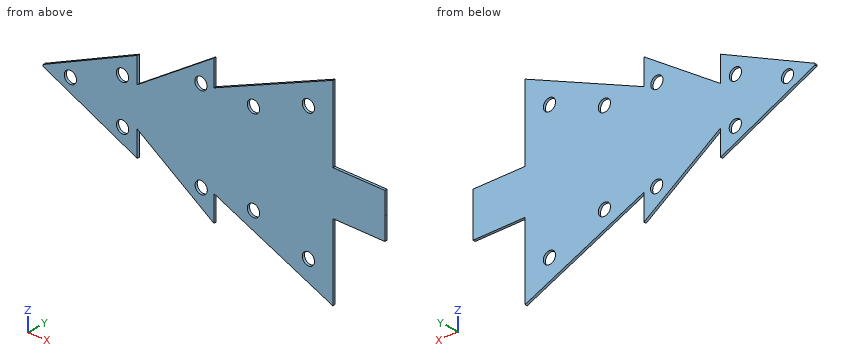
Autodesk Inventor part; units mm, degrees
ref_plane "YZ Plane" through (0, 0, 0) normal (1, 0, 0) x (0, 1, 0)
ref_plane "XZ Plane" through (0, 0, 0) normal (0, 1, 0) x (-1, 0, 0)
ref_plane "XY Plane" through (0, 0, 0) normal (0, 0, 1) x (1, 0, 0)
sketch "Sketch1" plane through (0, 0, 0) normal (0, 1, 0) x (-1, 0, 0)
  line L0 (-128.7932, -21.9318) -> (-128.8163, -31.0141)
  line L1 (11.205, -31.37) -> (11.2067, -30.7124)
  line L2 (11.2067, -30.7124) -> (-27.3951, -12.7346)
  line L3 (-27.3951, -12.7346) -> (-27.3951, -23.154)
  line L4 (-27.3951, -23.154) -> (-58.7933, -1.6646)
  line L5 (-58.7933, -1.6646) -> (-58.7933, -12.2738)
  line L6 (-58.7933, -12.2738) -> (-107.4995, 9.0183)
  line L7 (-107.4995, 9.0183) -> (-107.4995, -21.9859)
  line L8 (-107.4995, -21.9859) -> (-128.7932, -21.9318)
  line L9 (-128.8163, -40.0964) -> (-128.8163, -31.0141)
  line L10 (11.205, -31.37) -> (-27.3968, -49.3478)
  line L11 (-27.3968, -49.3478) -> (-27.3968, -38.9284)
  line L12 (-27.3968, -38.9284) -> (-58.795, -60.4178)
  line L13 (-58.795, -60.4178) -> (-58.795, -49.8086)
  line L14 (-58.795, -49.8086) -> (-107.5012, -71.1006)
  line L15 (-107.5012, -71.1006) -> (-107.5012, -40.0964)
  line L16 (-107.5012, -40.0964) -> (-128.8163, -40.0964)
  circle A0 centre (0, -31.0141) radius 2.5
  circle A1 centre (-21.3305, -22.0944) radius 2.5
  circle A2 centre (-53.494, -12.7333) radius 2.5
  circle A3 centre (-97.4998, -3.866) radius 2.5
  circle A4 centre (-75.0025, -12.7333) radius 2.5
  circle A5 centre (-21.3772, -40.48) radius 2.5
  circle A6 centre (-53.5879, -49.6775) radius 2.5
  circle A7 centre (-97.4998, -58.2188) radius 2.5
  circle A8 centre (-75.0025, -49.6775) radius 2.5
  point P0 (0, 0)
  dimension "d2" = 5
  dimension "d3" = 5
  dimension "d4" = 5
  dimension "d5" = 5
  dimension "d6" = 5
extrude "Extrusion1" add sketch "Sketch1" along normal blind 1
properties part number "Arbol"
Design review of the part built by this model. Coordinates are the model's own, in mm. Give positions to 0.01 mm unless a question says otherwise; leave off trailing zeros. Loops run counter-clockwise (first coordinate to the right, second up) from the corner with the lowest first, then second, coordinate; pieces in that order, holes last. Notation, with made-up numbers: (16.25, 64) -> (29.25, 64) arc R35 ccw to (29.25, 101) -> close; hole circle Ø7 at (47.25, 62.5). An arc over 180 degrees is marked (long way). One line per question, with ' | ' between items. Start each with the question number.
(1) We need section A-A (x = 54). State the section outline as (y, z) points, and give its area (3 significant figures).
(2) We need section B-B (y = 0.75). State how many separate pieces and enclosed holes the cut face has, and give its area (3 significant figures).
(3) We need section C-C (x = 0). State the section outline as (y, z) points, and give its area (3 significant figures).
(4) For line 1 (X direction, y = 0.8, z = -49); line 2 (Z direction, x = 23, y = 0.75); line 3 (Z direction, x = 52.5, y = 0.85), list the stretches that pass through material, from the lowest coordinate up.
(5) We need section D-D (z = -64.5). State the section outline as (x, y) points.
(6) Insertion check: P1, Ø4, axis at x = 53.49, z = -12.73, coming from the -Y side; P2, Ø0.5, axis at y = 0.5, z = -16, coming from the +X side. Each pin has a flat end and moves straight along its axis. Give the tip position at first contact, or say it passes through.
The answers:
1) outline: (0, -57.14) -> (1, -57.14) -> (1, -52.14) -> (0, -52.14) -> close; (0, -47.21) -> (1, -47.21) -> (1, -15.18) -> (0, -15.18) -> close; (0, -10.29) -> (1, -10.29) -> (1, -4.95) -> (0, -4.95) -> close | area: 42.4 mm^2
2) separate pieces: 1 | enclosed holes: 9 | area: 4,960 mm^2
3) outline: (0, -36.59) -> (1, -36.59) -> (1, -33.51) -> (0, -33.51) -> close; (0, -28.51) -> (1, -28.51) -> (1, -25.49) -> (0, -25.49) -> close | area: 6.10 mm^2
4) line 1: x = 26.65 to 27.4, 42.11 to 51.18, 55.99 to 72.6, 77.41 to 107.5 | line 2: z = -47.3 to -42.38, -38.58 to -23.96, -20.23 to -14.78 | line 3: z = -56.11 to -51.93, -47.43 to -15.03, -10.44 to -5.97
5) outline: (92.4, 0) -> (107.5, 0) -> (107.5, 1) -> (92.4, 1) -> close
6) P1: passes through | P2: stops at x = 107.5
